Can you work these out from the model? Positions are in its coordinate system, mm. A direction names the side the tool comes from. Coordinates: 2 decimals unless noted, no trailing zeros. Loops run counter-clockwise (first coordinate to the right, second up) from the corner with the lowest first, then second, coordinate; pieces in that order, holes last. Notation, with made-up numbers: M -33,12.5 L -14,12.5 A27 ccw -14,47.5 Z; hole C 10.25,5.5 d6. An arc over 180 degrees is marked long. Answer as a JSON object with one key per item and string values. Group by question number.
Item 1: We'd pull the mould along X, two halves only. Please class faces 3 (the flat face through (-88, 25, 2)), 4 (the flat face through (-186, 25, 1)): +X half, -X half, draft (parallel to the pull), parting line (faces both ways), or undercut.
Item 2: If I drill on line 1 (X direction, y = 27.5, z = 0.25), over which ranges is the centre line in solid material (lowest first)?
Item 3: Suppose I cut it at B-B (y = 21). Write out the boundary of the cut face in (x, z).
Item 4: Suppose I cut it at A-A (z = 0.55). Write out the boundary of the cut face in (x, y), then the cut area to 3 significant figures.
Item 5: Which directions (+Z, -Z, +X, -X, +Y, -Y) give clear straight access to the entire face, cutting with the end or side of a thin tool? Please do faces 1 (the flat face through (12, 25, 1)), 2 (the flat face through (-88, 25, 0)).
Autodesk Inventor part; units mm, degrees
ref_plane "YZ Plane" through (0, 0, 0) normal (1, 0, 0) x (0, 1, 0)
ref_plane "XZ Plane" through (0, 0, 0) normal (0, 1, 0) x (-1, 0, 0)
ref_plane "XY Plane" through (0, 0, 0) normal (0, 0, 1) x (1, 0, 0)
sketch "스케치1" plane through (0, 0, 0) normal (0, 0, 1) x (1, 0, 0)
  line L0 (-190, 35) -> (16, 35)
  line L1 (16, 35) -> (16, 15)
  line L2 (16, 15) -> (-190, 15)
  line L3 (-190, 15) -> (-190, 35)
  point P0 (0, 0)
  dimension "d0" = 206
  dimension "d1" = 20
extrude "돌출1" add sketch "스케치1" along normal blind 2
sketch "스케치2" plane through (0, 0, 0) normal (0, 0, -1) x (-1, 0, 0)
  line L0 (-16, 35) -> (190, 35)
  line L1 (190, 15) -> (-16, 15)
  line L2 (-15, 35) -> (-9.6, 35)
  line L3 (-9.6, 35) -> (-9.6, 15)
  line L4 (-9.6, 15) -> (-15, 15)
  line L5 (-15, 15) -> (-15, 35)
  line L6 (189, 35) -> (183.6, 35)
  line L7 (183.6, 35) -> (183.6, 15)
  line L8 (183.6, 15) -> (189, 15)
  line L9 (189, 15) -> (189, 35)
  line L10 (190, 15) -> (190, 35)
  line L11 (-16, 35) -> (-16, 15)
  point P0 (0, 0)
  dimension "d4" = 5.4
  dimension "d5" = 5.4
  dimension "d6" = 1
  dimension "d7" = 1
extrude "돌출2" cut sketch "스케치2" against normal blind 1 contours L0 L3 L1 L5 | L0 L9 L1 L7
properties part number "앞판_위" material "알루미늄 6061"
From the geometry:
{
 "1": {"face 3": "draft", "face 4": "undercut"},
 "2": {"line 1": "-190 to -189, -183.6 to 9.6, 15 to 16"},
 "3": {"outline": "M -190,0 L -189,0 L -189,1 L -183.6,1 L -183.6,0 L 9.6,0 L 9.6,1 L 15,1 L 15,0 L 16,0 L 16,2 L -190,2 Z"},
 "4": {"outline": "M -190,15 L -189,15 L -189,35 L -190,35 Z; M -183.6,15 L 9.6,15 L 9.6,35 L -183.6,35 Z; M 15,15 L 16,15 L 16,35 L 15,35 Z", "area": "3,900 mm2"},
 "5": {"face 1": "-Z, +Y, -Y", "face 2": "-Z, +X, -X, +Y, -Y"}
}
